The figure shows three views and two pictorial views of one solid part (mm, origin at its lowest corner). Answer the questions. A direction names the side the tool comes from. Coordinates: 2 decimals unless noted, no trailing zeros. Loops run counter-clockwise (first coordinate to the right, second up) from the corner with the lowest first, then second, coordinate; pieces in that order, holes last.
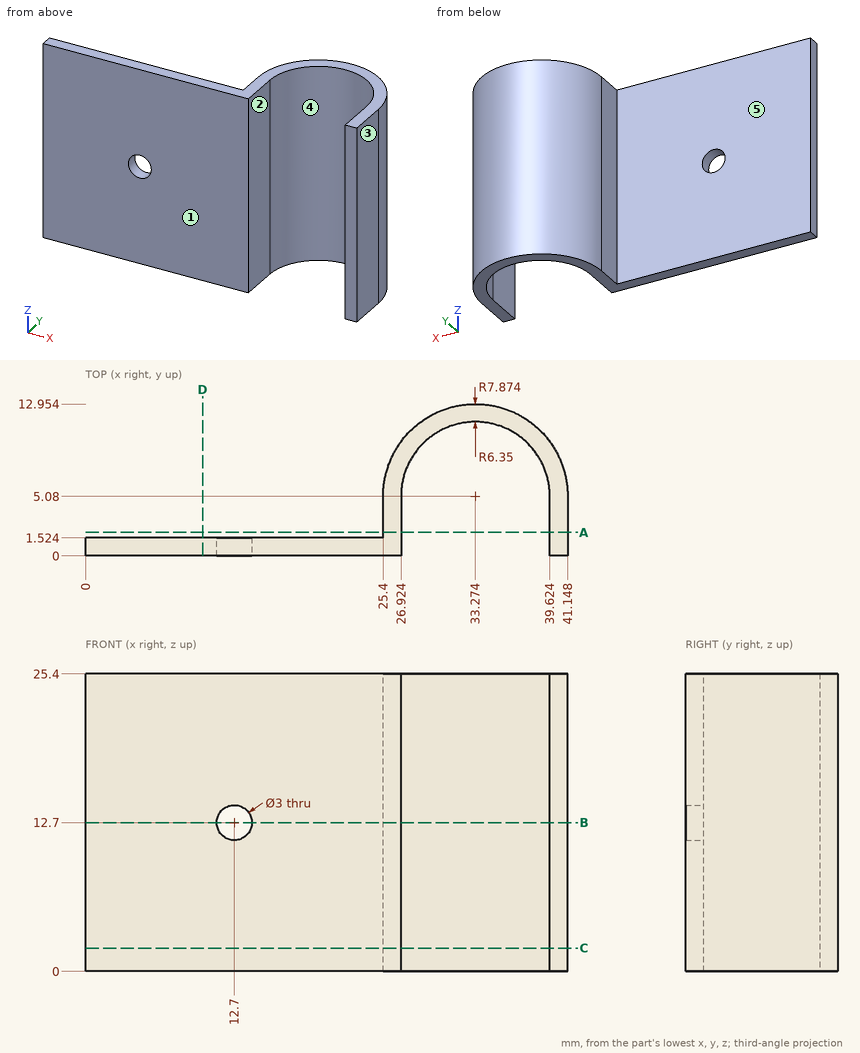
Q1. Straight lines are drawn through the part: probe 1 along Z at (x, y) = (12.7, 0.7); probe 2 along X at (y, z) = (0.85, 12.7); probe 3 along X at (y, z) = (3.25, 16). For each, find the intervals that lie inside material, in ascending order.
Findings below:
probe 1: z = 0 to 11.2, 14.2 to 25.4
probe 2: x = 0 to 11.2, 14.2 to 26.92, 39.62 to 41.15
probe 3: x = 25.4 to 26.92, 39.62 to 41.15
Q2. Which of the six approach directions +Z, -Z, +X, -X, +Y, -Y give full straight-line access (tool end or side, diameter ignored) to the marked faces 1 and 2?
Findings below:
face 1: +Z, -Z, +X, -X, -Y
face 2: +Z, -Z, -Y
Q3. A cutting plane is placed at A-A (y = 2). Give the vertices of the cut face in (x, z).
Findings below:
outline: (25.4, 0) - (26.92, 0) - (26.92, 25.4) - (25.4, 25.4) - close; (39.62, 0) - (41.15, 0) - (41.15, 25.4) - (39.62, 25.4) - close
Q4. Flat-ended cylindrical pins translate along their axes: pin 1 Ø2 at (y, z) = (7.5, 22) entering from -X; pin 2 Ø12 at (x, z) = (18, 22) entering from +Y; pin 3 Ø3 at (y, z) = (10.5, 12) entering from +X; pin 4 Ø1.5 at (y, z) = (1.5, 10) entering from -X. Find the tip coordinate at first contact, or state that the pin passes through.
Findings below:
pin 1: stops at x = 25.53
pin 2: stops at y = 1.52
pin 3: stops at x = 40.1
pin 4: stops at x = 0
Q5. Determine the mould class of the marked faces 3, 4 and 5 for opening direction X: +X half, -X half, draft (parallel to the pull), parting line (faces both ways), or undercut.
Findings below:
face 3: +X half
face 4: undercut
face 5: draft
Q6. A cutting plane is placed at B-B (z = 12.7). Give the vertices of the cut face in (x, y).
Findings below:
outline: (0, 0) - (11.2, 0) - (11.2, 1.52) - (0, 1.52) - close; (14.2, 0) - (26.92, 0) - (26.92, 5.08) arc R6.35 cw to (39.62, 5.08) - (39.62, 0) - (41.15, 0) - (41.15, 5.08) arc R7.87 ccw to (25.4, 5.08) - (25.4, 1.52) - (14.2, 1.52) - close
Q7. A cutting plane is placed at C-C (z = 2). Give the vertices of the cut face in (x, y), then the cut area to 3 significant figures.
Findings below:
outline: (0, 0) - (26.92, 0) - (26.92, 5.08) arc R6.35 cw to (39.62, 5.08) - (39.62, 0) - (41.15, 0) - (41.15, 5.08) arc R7.87 ccw to (25.4, 5.08) - (25.4, 1.52) - (0, 1.52) - close
area: 88.2 mm2
Q8. A cutting plane is placed at D-D (x = 10). Give the vertices of the cut face in (y, z).
Findings below:
outline: (0, 0) - (1.52, 0) - (1.52, 25.4) - (0, 25.4) - close
